Source: CAD feature listing. Evaluate the final solid. Frame: model axes, mm. Coordinates: 2 decimals unless noted, no trailing zeros. Order: outer loops, then holes, each group sorted by start corner. A loop starts at its lowest first (then second) coordinate and runs counter-clockwise, first axis right, second up.
```python
from build123d import *

# Parameters (mm, degrees)
F1_DEPTH = 6.35
F3_DEPTH = 25.4
F5_DEPTH = 25.4


with BuildPart() as f1:
    # F0 (on Top) → F1 (new body)
    with BuildSketch(Plane.XY):
        with BuildLine():
            Line((113.9825, 84.1375), (-113.9825, 84.1375))
            ThreePointArc((-113.9825, 84.1375), (-117.574602, 82.649602), (-119.0625, 79.0575))
            Line((-119.0625, 79.0575), (-119.0625, -79.0575))
            ThreePointArc((-119.0625, -79.0575), (-117.574602, -82.649602), (-113.9825, -84.1375))
            Line((-113.9825, -84.1375), (113.9825, -84.1375))
            ThreePointArc((113.9825, -84.1375), (117.574602, -82.649602), (119.0625, -79.0575))
            Line((119.0625, -79.0575), (119.0625, 79.0575))
            ThreePointArc((119.0625, 79.0575), (117.574602, 82.649602), (113.9825, 84.1375))
        make_face()
    extrude(amount=F1_DEPTH)

    # F2 (on face) → F3 (cut)
    with BuildSketch(Plane.XY.offset(6.35)):
        Polygon((22.606, 44.54207), (0, 44.54207), (-22.606, 44.54207), (-67.14807, 0), (-67.14807, -44.958), (-22.19007, -44.958), (-22.19007, 0), (0, 0), (22.19007, 0), (22.19007, -44.958), (67.14807, -44.958), (67.14807, 0), align=None)
    extrude(amount=-F3_DEPTH, mode=Mode.SUBTRACT)

    # F4 (on face) → F5 (cut)
    with BuildSketch(Plane.XY.offset(6.35)):
        with BuildLine():
            ThreePointArc((-22.805899, 45.81207), (-23.107224, 45.752133), (-23.362675, 45.581446))
            Line((-23.362675, 45.581446), (-68.187446, 0.756675))
            ThreePointArc((-68.187446, 0.756675), (-68.358133, 0.501224), (-68.41807, 0.199899))
            Line((-68.41807, 0.199899), (-68.41807, -45.4406))
            ThreePointArc((-68.41807, -45.4406), (-68.187446, -45.997376), (-67.63067, -46.228))
            Line((-67.63067, -46.228), (-21.70747, -46.228))
            ThreePointArc((-21.70747, -46.228), (-21.150694, -45.997376), (-20.92007, -45.4406))
            Line((-20.92007, -45.4406), (-20.92007, -2.0574))
            ThreePointArc((-20.92007, -2.0574), (-20.689446, -1.500624), (-20.13267, -1.27))
            Line((-20.13267, -1.27), (20.13267, -1.27))
            ThreePointArc((20.13267, -1.27), (20.689446, -1.500624), (20.92007, -2.0574))
            Line((20.92007, -2.0574), (20.92007, -45.4406))
            ThreePointArc((20.92007, -45.4406), (21.150694, -45.997376), (21.70747, -46.228))
            Line((21.70747, -46.228), (67.63067, -46.228))
            ThreePointArc((67.63067, -46.228), (68.187446, -45.997376), (68.41807, -45.4406))
            Line((68.41807, -45.4406), (68.41807, 0.199899))
            ThreePointArc((68.41807, 0.199899), (68.358133, 0.501224), (68.187446, 0.756675))
            Line((68.187446, 0.756675), (23.362675, 45.581446))
            ThreePointArc((23.362675, 45.581446), (23.107224, 45.752133), (22.805899, 45.81207))
            Line((22.805899, 45.81207), (-22.805899, 45.81207))
        make_face()
    extrude(amount=-F5_DEPTH, mode=Mode.SUBTRACT)


solid = f1.part
```
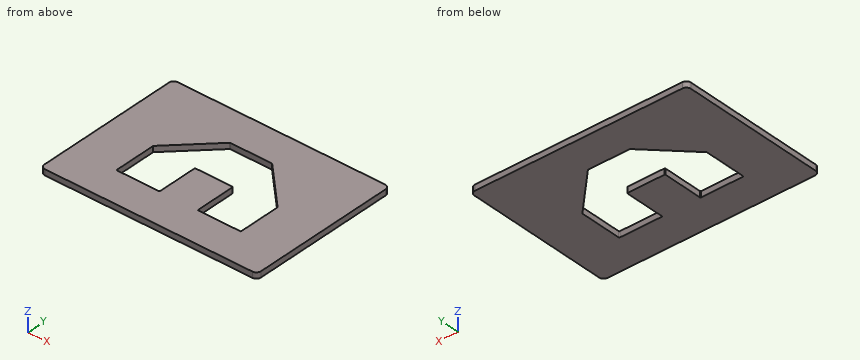
Q1. Section query D-D on y = 10. Output: boundary loops of the cut face in (x, z).
Solutions:
outline: (-119.06, 0) - (-58.94, 0) - (-58.94, 6.35) - (-119.06, 6.35) - close; (58.94, 0) - (119.06, 0) - (119.06, 6.35) - (58.94, 6.35) - close
Q2. Section query A-A on x = 12. Output: boundary loops of the cut face in (y, z), plus the area to 3 significant figures.
Solutions:
outline: (-84.14, 0) - (-1.27, 0) - (-1.27, 6.35) - (-84.14, 6.35) - close; (45.81, 0) - (84.14, 0) - (84.14, 6.35) - (45.81, 6.35) - close
area: 770 mm2
Q3. Section query B-B on y = -10.5. Output: boundary loops of the cut face in (x, z).
Solutions:
outline: (-119.06, 0) - (-68.42, 0) - (-68.42, 6.35) - (-119.06, 6.35) - close; (-20.92, 0) - (20.92, 0) - (20.92, 6.35) - (-20.92, 6.35) - close; (68.42, 0) - (119.06, 0) - (119.06, 6.35) - (68.42, 6.35) - close
Q4. Section query C-C on z = 3. Output: boundary loops of the cut face in (x, y), plus the area to 3 significant figures.
Solutions:
outline: (-119.06, -79.06) arc R5.08 ccw to (-113.98, -84.14) - (113.98, -84.14) arc R5.08 ccw to (119.06, -79.06) - (119.06, 79.06) arc R5.08 ccw to (113.98, 84.14) - (-113.98, 84.14) arc R5.08 ccw to (-119.06, 79.06) - close; hole (-68.42, -45.44) arc R0.79 ccw to (-67.63, -46.23) - (-21.71, -46.23) arc R0.79 ccw to (-20.92, -45.44) - (-20.92, -2.06) arc R0.79 cw to (-20.13, -1.27) - (20.13, -1.27) arc R0.79 cw to (20.92, -2.06) - (20.92, -45.44) arc R0.79 ccw to (21.71, -46.23) - (67.63, -46.23) arc R0.79 ccw to (68.42, -45.44) - (68.42, 0.2) arc R0.79 ccw to (68.19, 0.76) - (23.36, 45.58) arc R0.79 ccw to (22.81, 45.81) - (-22.81, 45.81) arc R0.79 ccw to (-23.36, 45.58) - (-68.19, 0.76) arc R0.79 ccw to (-68.42, 0.2) - close
area: 31,400 mm2
Q5. Material intervals for line 1 along X through (y, z) = (-21.5, 3.75); line 2 along Y through (x, z) = (10, 3); line 3 along Y through (x, z) = (43, 4.25), sorted ascending.
Solutions:
line 1: x = -119.06 to -68.42, -20.92 to 20.92, 68.42 to 119.06
line 2: y = -84.14 to -1.27, 45.81 to 84.14
line 3: y = -84.14 to -46.23, 25.94 to 84.14
